For this review, take the finished solid that the model builds, in its own axes (mm). Face numbers are marked on the shaded views. A direction names the side the tool comes from. Round coordinates to 2 decimals unless told otherwise and drop trailing zeros. Loops run counter-clockwise (first coordinate to the right, second up) from the corner with the lowest first, then second, coordinate; pieces in that order, holes last. Notation, with made-up numbers: (67, -6.5) -> (123, -6.5) arc R10 cw to (123, 0.5) -> close; hole circle Ø3 at (-36.5, 83.5). An arc over 180 degrees is marked (long way). Write each question's results on one line, items separated by ' | '.
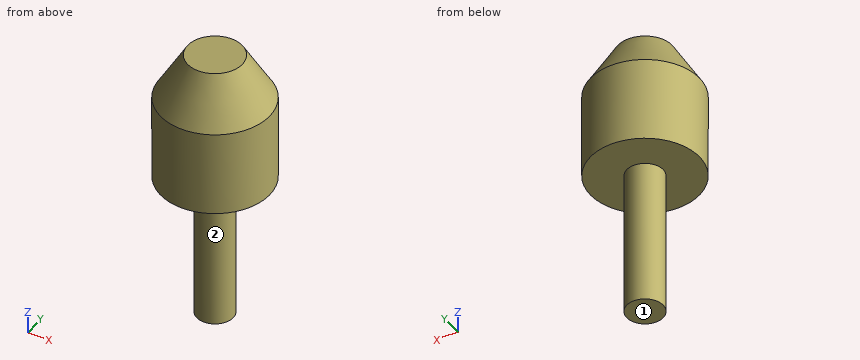
```python
from build123d import *

# Parameters (mm, degrees)
SKETCH_1_R      = 2
EXTRUDE_1_DEPTH = 16
SKETCH_2_R      = 6
EXTRUDE_2_DEPTH = 14.3


with BuildPart() as part:
    # 草图1 → 凸台-拉伸1 (new body)
    with BuildSketch(Plane.XY):
        Circle(SKETCH_1_R)
    extrude(amount=EXTRUDE_1_DEPTH)

    # 草图2 → 凸台-拉伸2 (add)
    with BuildSketch(Plane.XY.offset(16)):
        Circle(SKETCH_2_R)
    extrude(amount=EXTRUDE_2_DEPTH)

    # 草图3 → 切除-旋转2 (revolve, cut)
    with BuildSketch(Plane(origin=(0, 0, 0), x_dir=(1, 0, 0), z_dir=(0, 1, 0))):
        Polygon((-3, -30.3), (-6, -25.3), (-6, -30.3), align=None)
    revolve(axis=Axis((0, 0, 0), (0, 0, 1)), mode=Mode.SUBTRACT)


solid = part.part
```
1. Consider section C-C (z = 28). State the section outline as (x, y) points.
Values found:
outline: circle Ø8.76 at (0, 0)
2. Consider section D-D (z = 8.5). State the section outline as (x, y) points, plus the area to 3 significant figures.
Values found:
outline: circle Ø4 at (0, 0) | area: 12.6 mm2
3. Tool access review of the marked faces 1 and 2: name each direction out of +Z, -Z, +X, -X, +Y, -Y from which nothing blocks a thin tool from reaching the whole face with its end or side.
Values found:
face 1: -Z, +X, -X, +Y, -Y | face 2: -Z
4. To check wall thickness, follow probe 1 along X at (y, z) = (0.25, 23.5); probe 2 along Z at (x, y) = (1.5, -2.5); probe 3 along X at (y, z) = (0.5, 26). State the ranges of each line that lie inside material, in increasing order.
Values found:
probe 1: x = -5.99 to 5.99 | probe 2: z = 16 to 30.3 | probe 3: x = -5.56 to 5.56
5. For pin 1 (6 mm diameter, centred on y = 2.5, z = 5.5, fed in from +X); pin 2 (4 mm diameter, centred on x = -4, y = 4, fed in from -Z), all flat-tipped, find the tip position at first contact; note any pin that passes through.
Values found:
pin 1: stops at x = 2 | pin 2: stops at z = 16
6. Consider section A-A (y = 0). State the section outline as (x, z) points.
Values found:
outline: (-6, 16) -> (-2, 16) -> (-2, 0) -> (2, 0) -> (2, 16) -> (6, 16) -> (6, 25.3) -> (3, 30.3) -> (-3, 30.3) -> (-6, 25.3) -> close
